from build123d import *

# Parameters (mm, degrees)
F0_R     = 3.1
F1_DEPTH = 20.5
F3_DEPTH = 5.6
F4_W     = 6.3
F4_H     = 0.8
F5_DEPTH = 9
F6_SIZE  = 1


with BuildPart() as f1:
    # F0 (on Top) → F1 (new body)
    with BuildSketch(Plane.XY):
        with BuildLine():
            Line((-22.95, -26.75), (22.95, -26.75))
            ThreePointArc((22.95, -26.75), (25.637006, -25.637006), (26.75, -22.95))
            Line((26.75, -22.95), (26.75, 22.95))
            ThreePointArc((26.75, 22.95), (25.637006, 25.637006), (22.95, 26.75))
            Line((22.95, 26.75), (-22.95, 26.75))
            ThreePointArc((-22.95, 26.75), (-25.637006, 25.637006), (-26.75, 22.95))
            Line((-26.75, 22.95), (-26.75, -22.95))
            ThreePointArc((-26.75, -22.95), (-25.637006, -25.637006), (-22.95, -26.75))
        make_face()
        Circle(F0_R, mode=Mode.SUBTRACT)
    extrude(amount=F1_DEPTH)

    # F2 (on face) → F3 (join)
    with BuildSketch(Plane.XY.offset(20.5)):
        Polygon((4.3, 13.718882), (4.3, 17.281118), (1.781118, 19.8), (-1.781118, 19.8), (-4.3, 17.281118), (-4.3, 13.718882), (-1.781118, 11.2), (1.781118, 11.2), align=None)
    extrude(amount=F3_DEPTH)

    # F4 (on face) → F5 (join)
    with BuildSketch(Plane.XY.offset(20.5)):
        with Locations((-15.55, -20.45)):
            Rectangle(F4_W, F4_H)
        with Locations((15.55, -20.45)):
            Rectangle(F4_W, F4_H)
    extrude(amount=F5_DEPTH)

    # F6
    f6_edges = [f1.edges().sort_by_distance(p)[0] for p in [
        (-18.7, -20.45, 29.5),
        (-12.4, -20.45, 29.5),
        (12.4, -20.45, 29.5),
        (18.7, -20.45, 29.5),
    ]]
    chamfer(f6_edges, length=F6_SIZE)


solid = f1.part
Could you check a few things on this model? Use its own coordinates, in mm. A direction names the side the tool comes from. Coordinates: 2 decimals unless noted, no trailing zeros. Order: outer loops, then holes, each group sorted by start corner. A loop starts at its lowest first (then second) coordinate and runs counter-clockwise, first axis right, second up.
Q1. Suppose I cut it at A-A on y = 0. Please give me the cut outline in (x, z).
Q2. Suppose I cut it at C-C on x = -14.5. Please give me the cut outline in (y, z).
Q3. Which directions (+Z, -Z, +X, -X, +Y, -Y) give clear straight access to the entire face, cutting with the end or side of a thin tool? Please do faces 1 (the flat face through (3.06, 18.52, 23.26)), 2 (the flat face through (-4.3, 16, 23)), 3 (the flat face through (0, 19.8, 23)).
Q4. Will these pins go through, and if not, where does the flat tip stop? pin 1 (10 mm diameter, centred on y = -16, z = 26.5, fed in from -X); pin 2 (7 mm diameter, centred on x = 14, z = 26, fed in from +Y); pin 3 (5 mm diameter, centred on x = 16.5, z = 25, fed in from -Y).
Q5. Please list where these lines run through material, in increasing order: L1, parallel to Y at x = 0, z = 13; L2, parallel to Z at x = 7, y = 12; L3, parallel to Y at x = 17.5, z = 27.5.
Q6. Suppose I cut it at D-D on y = 9. Please give me the cut outline in (x, z), and give its area (3 significant figures).
Q7. Suppose I cut it at B-B on x = 0. Please give me the cut outline in (y, z).
Answer:
1. outline: (-26.75, 0) - (-3.1, 0) - (-3.1, 20.5) - (-26.75, 20.5) - close; (3.1, 0) - (26.75, 0) - (26.75, 20.5) - (3.1, 20.5) - close
2. outline: (-26.75, 0) - (26.75, 0) - (26.75, 20.5) - (-20.05, 20.5) - (-20.05, 29.5) - (-20.85, 29.5) - (-20.85, 20.5) - (-26.75, 20.5) - close
3. face 1: +Z, +X, +Y
3. face 2: +Z, -X, +Y, -Y
3. face 3: +Z, +X, -X, +Y
4. pin 1: stops at x = -18.7
4. pin 2: stops at y = -20.05
4. pin 3: stops at y = -20.85
5. L1: y = -26.75 to -3.1, 3.1 to 26.75
5. L2: z = 0 to 20.5
5. L3: y = -20.85 to -20.05
6. outline: (-26.75, 0) - (26.75, 0) - (26.75, 20.5) - (-26.75, 20.5) - close
6. area: 1,100 mm2
7. outline: (-26.75, 0) - (-3.1, 0) - (-3.1, 20.5) - (-26.75, 20.5) - close; (3.1, 0) - (26.75, 0) - (26.75, 20.5) - (19.8, 20.5) - (19.8, 26.1) - (11.2, 26.1) - (11.2, 20.5) - (3.1, 20.5) - close
